Autodesk Inventor part; units mm, degrees
ref_plane "YZ Plane" through (0, 0, 0) normal (1, 0, 0) x (0, 1, 0)
ref_plane "XZ Plane" through (0, 0, 0) normal (0, 1, 0) x (-1, 0, 0)
ref_plane "XY Plane" through (0, 0, 0) normal (0, 0, 1) x (1, 0, 0)
sketch "Sketch1" plane through (0, 0, 0) normal (0, 0, 1) x (1, 0, 0)
  circle A0 centre (10.538, 13.901) radius 1.5
  circle A1 centre (-14.3574, -8.5148) radius 1.5
  line L0 (-15.1125, -4.8626) -> (-12.2879, -5.0107)
  line L1 (-15.1125, -4.8626) -> (-18.0851, -7.5392)
  line L2 (-15.5871, -15.1392) -> (-18.0851, -7.5392)
  line L3 (16.4403, 13.6984) -> (-15.5871, -15.1392)
  line L4 (16.4403, 13.6984) -> (10.1865, 17.9166)
  line L5 (10.1865, 17.9166) -> (7.2139, 15.2401)
  line L6 (7.0659, 12.4156) -> (7.2139, 15.2401)
  line L7 (7.0659, 12.4156) -> (7.6141, 11.8066)
  arc A2 (7.4661, 8.9821) -> (7.6141, 11.8066) centre (6.1278, 10.4684) ccw
  line L8 (-8.9151, -5.7676) -> (7.4661, 8.9821)
  arc A3 (-11.7396, -5.6196) -> (-8.9151, -5.7676) centre (-10.2534, -4.2813) ccw
  line L9 (-11.7396, -5.6196) -> (-12.2879, -5.0107)
  circle A4 centre (-17.5227, 24.7135) radius 1.5
  circle A5 centre (-17.5227, 24.7135) radius 3
  circle A6 centre (-17.5227, 24.7135) radius 6
  line L10 (-18.0851, -7.5392) -> (-23.4365, 23.7005)
  line L11 (10.1865, 17.9166) -> (-14.8998, 30.1099)
  line L12 (-15.1125, -4.8626) -> (-19.1917, 18.9503)
  line L13 (7.2139, 15.2401) -> (-11.5335, 24.3523)
  point P0 (0, 0)
  dimension "d0" = 6
  dimension "d1" = 12
extrude "Extrusion1" add sketch "Sketch1" along normal blind 2 contours L0 L9 A3 L8 A2 L7 L6 L5 L4 L3 L2 L1 | L1 L10 A6 L12 | A6 | A6 L11 L5 L13
chamfer "Chamfer1" distance 3 angle 45 2 edges at (16.4403, 13.6984, 1) (-15.5871, -15.1392, 1)
sketch "Sketch2" plane through (0, 0, 2) normal (0, 0, 1) x (1, 0, 0)
  line L0 (-13.3576, -13.1318) -> (-16.5238, -12.2892)
  line L1 (-13.3576, -13.1318) -> (14.2108, 11.691)
  line L2 (13.9532, 15.376) -> (14.2108, 11.691)
  line L3 (13.9532, 15.376) -> (10.1865, 17.9166)
  line L4 (10.1865, 17.9166) -> (-14.8998, 30.1099)
  arc A0 (-14.8998, 30.1099) -> (-23.4365, 23.7005) centre (-17.5227, 24.7135) ccw
  line L5 (-23.4365, 23.7005) -> (-18.0851, -7.5392)
  line L6 (-18.0851, -7.5392) -> (-16.5238, -12.2892)
  circle A1 centre (-17.5227, 24.7135) radius 3
  circle A2 centre (10.538, 13.901) radius 1.5
  circle A3 centre (-14.3574, -8.5148) radius 1.5
  line L7 (-15.1125, -4.8626) -> (-19.1917, 18.9503)
  arc A4 (-19.1917, 18.9503) -> (-11.5335, 24.3523) centre (-17.5227, 24.7135) ccw
  line L8 (-11.5335, 24.3523) -> (7.2139, 15.2401)
  line L9 (7.2139, 15.2401) -> (7.0659, 12.4156)
  line L10 (7.0659, 12.4156) -> (7.6141, 11.8066)
  arc A5 (7.4661, 8.9821) -> (7.6141, 11.8066) centre (6.1278, 10.4684) ccw
  line L11 (7.4661, 8.9821) -> (-8.9151, -5.7676)
  arc A6 (-11.7396, -5.6196) -> (-8.9151, -5.7676) centre (-10.2534, -4.2813) ccw
  line L12 (-11.7396, -5.6196) -> (-12.2879, -5.0107)
  line L13 (-12.2879, -5.0107) -> (-15.1125, -4.8626)
  circle A7 centre (-14.3574, -8.5148) radius 1.5
  circle A8 centre (-14.3574, -8.5148) radius 1
  circle A9 centre (10.538, 13.901) radius 1
  point P0 (0, 0)
  dimension "d7" = 2
  dimension "d8" = 2
extrude "Extrusion2" add sketch "Sketch2" against normal blind 2 contours A2 | A3
fillet "Fillet1" radius 1 2 edges at (-19.1917, 18.9503, 1) (-11.5335, 24.3523, 1)
properties part number "stand_3"
Can you work these out from the model? Positions are in its coordinate system, mm. A direction names the side the tool comes from. Round coordinates to 2 decimals unless told otherwise and drop trailing zeros. Loops run counter-clockwise (first coordinate to the right, second up) from the corner with the lowest first, then second, coordinate; pieces in that order, holes last. Notation, with made-up numbers: (-38, 68) - (2, 68) arc R20 cw to (2, 76) - close; hole circle Ø11 at (32.25, -23). An arc over 180 degrees is marked (long way). Answer in a Markdown table with one row per item. Add a question column.
Q1. I need wall thicknesses on L1, parallel to X at y = 13.5, z = 0.95; L2, parallel to X at y = 22.5, z = 0.8; L3, parallel to X at y = 15.5, z = 1. Which ranges of each line are inside material? Lowest first, please.
Q2. Which directions (+Z, -Z, +X, -X, +Y, -Y) give clear straight access to the entire face, cutting with the end or side of a thin tool? Please do faces 4 (the cylindrical face through (-11.172, 23.785, 1.014)), 5 (the flat face through (0.62, -0.547, 0.986)).
Q3. We'd pull the mould along X, two halves only. Please class faces 1 (the flat face through (-20.723, 7.862, 0.986)), 2 (the cylindrical face through (-13.988, 19.865, 0.986)), 3 (the flat face through (-2.181, 23.928, 0.986)): pulls with the +X half, pulls with the -X half, needs draft (parallel to the pull), parting line crosses it, or undercut.
Q4. I want a section at C-C on z = 1.4. List the corners of the cut face in (x, y) for me.
Q5. I want a section at B-B on x = -6.5. List the corners of the cut face in (y, z) for me.
Q6. I want a section at D-D on y = 9.5. List the corners of the cut face in (x, z) for me, and give its area (3 significant figures).
Q7. For pin 1 Ø1 at (x, z) = (7, 0.5) entering from +Y, with a flat end and sliding along its axis, tell me the tip position at first contact or that it passes through.
Q8. I want a section at A-A on y = 22.5. List the corners of the cut face in (x, z) for me.
A:
| question | item | result |
|---|---|---|
| 1 | L1 | -21.69 to -18.26, 7.12 to 9.62, 11.45 to 14.08 |
| 1 | L2 | -23.23 to -19.55, -15.5 to -11.95, -7.72 to 0.76 |
| 1 | L3 | -22.03 to -18.6, 6.68 to 13.77 |
| 2 | face 4 | +Z, -Z |
| 2 | face 5 | +Z, -Z, +X, -Y |
| 3 | face 1 | pulls with the -X half |
| 3 | face 2 | undercut |
| 3 | face 3 | pulls with the +X half |
| 4 | outline | (-23.44, 23.7) - (-18.09, -7.54) - (-16.52, -12.29) - (-13.36, -13.13) - (14.21, 11.69) - (13.95, 15.38) - (10.19, 17.92) - (-14.9, 30.11) arc R6 ccw to start; hole circle Ø6 at (-17.52, 24.71); hole (-18.95, 17.56) - (-15.11, -4.86) - (-12.29, -5.01) - (-11.74, -5.62) arc R2 ccw to (-8.92, -5.77) - (7.47, 8.98) arc R2 ccw to (7.61, 11.81) - (7.07, 12.42) - (7.21, 15.24) - (-10.33, 23.77) arc R1 ccw to (-11.73, 23.13) arc R6 cw to (-17.9, 18.73) arc R1 ccw to start; hole circle Ø2 at (-14.36, -8.51); hole circle Ø2 at (10.54, 13.9) |
| 5 | outline | (-6.96, 0) - (-3.59, 0) - (-3.59, 2) - (-6.96, 2) - close; (21.91, 0) - (26.03, 0) - (26.03, 2) - (21.91, 2) - close |
| 6 | outline | (-21, 0) - (-17.57, 0) - (-17.57, 2) - (-21, 2) - close; (7.88, 0) - (11.78, 0) - (11.78, 2) - (7.88, 2) - close |
| 6 | area | 14.7 mm^2 |
| 7 | pin 1 | y = 19.71 |
| 8 | outline | (-23.23, 0) - (-19.55, 0) - (-19.55, 2) - (-23.23, 2) - close; (-15.5, 0) - (-11.95, 0) - (-11.95, 2) - (-15.5, 2) - close; (-7.72, 0) - (0.76, 0) - (0.76, 2) - (-7.72, 2) - close |
